Build history of the part. All positions in model axes, mm. A direction names the side the tool comes from. Coordinates: 2 decimals unless noted, no trailing zeros. Loops run counter-clockwise (first coordinate to the right, second up) from the corner with the lowest first, then second, coordinate; pieces in that order, holes last. Notation, with made-up numbers: (70, 23.5) -> (91, 23.5) arc R12 ccw to (91, 32.5) -> close; hole circle Ø4 at (38, 14.5). An arc over 180 degrees is marked (long way). One line per item, written item: value. Start each with the question number.
```python
from build123d import *

# Parameters (mm, degrees)
F0_W     = 55
F0_H     = 70
F1_DEPTH = 33
F2_T     = -3
F3_W     = 5
F3_H     = 30
F4_DEPTH = 55
F5_R     = 5.5
F6_DEPTH = 3
F7_R     = 1.65
F8_DEPTH = 3


with BuildPart() as f1:
    # F0 (on Top) → F1 (new body)
    with BuildSketch(Plane.XY):
        with Locations((27.5, 35)):
            Rectangle(F0_W, F0_H)
    extrude(amount=F1_DEPTH)

    # F2
    f2_openings = [f1.faces().sort_by_distance(p)[0] for p in [
        (27.5, 35, 0),
    ]]
    offset(amount=F2_T, openings=f2_openings)

    # F3 (on face) → F4 (cut, through all)
    with BuildSketch(Plane.YZ.offset(55)):
        with Locations((67.5, 15)):
            Rectangle(F3_W, F3_H)
    extrude(amount=-F4_DEPTH, mode=Mode.SUBTRACT)

    # F5 (on face) → F6 (cut, through all)
    with BuildSketch(Plane.XZ):
        with Locations((10, 11)):
            Circle(F5_R)
    extrude(amount=-F6_DEPTH, mode=Mode.SUBTRACT)

    # F7 (on face) → F8 (cut, through all)
    with BuildSketch(Plane.XY.offset(33)):
        with Locations((27.5, 67.5)):
            Circle(F7_R)
    extrude(amount=-F8_DEPTH, mode=Mode.SUBTRACT)


solid = f1.part
```
Item 1: Band-saw the part on D-D, the plane x = 43. List the corners of the cut face in (y, z).
Item 2: Tool access for faces 4 (the face through (27, 0, 16)), 5 (the face through (3, 34, 15)), 6 (the face through (54, 65, 15)): list every direction of +Z, -Z, +X, -X, +Y, -Y with a clear straight run to the whole face (end or side of a thin tool).
Item 3: Drop flat-ended pins along their axis: pin 1 Ø0.9 at (x, z) = (2, 18.5) entering from +Y; pin 2 Ø1 at (x, z) = (48, 15.5) entering from +Y; pin 3 Ø10 at (x, y) = (41.5, 40) entering from -Z. Give the stop position or say it passes through.
Item 4: Band-saw the part on C-C, the plane z = 17.5. List the corners of the cut face in (x, y), and give its area (3 significant figures).
Item 5: Probe probe 1 along X at (y, z) = (34, 4); probe 2 along Z at (x, y) = (10, 0.6); probe 3 along Z at (x, y) = (10, 10). List the from-to ranges inside material, lowest first.
Item 6: Band-saw the part on A-A, the plane x = 27.5. List the corners of the cut face in (y, z), and give its area (3 significant figures).
Item 7: Two-plate mould, pull along Y, no slides. Class faces 1 (the face through (27.1, 65.9, 31.5)), 2 (the face through (15.08, 1.48, 8.89)), 3 (the face through (2, 65, 15)): +Y half, -Y half, draft (parallel to the pull), parting line (faces both ways), or undercut.
Item 8: Band-saw the part on B-B, the plane y = 67.5. List the corners of the cut face in (x, z).
Worked out:
1. outline: (0, 0) -> (3, 0) -> (3, 30) -> (70, 30) -> (70, 33) -> (0, 33) -> close
2. face 4: +Z, -Z, +X, -X, -Y
2. face 5: -Z, +Y
2. face 6: -Z, +X, -X, +Y
3. pin 1: stops at y = 65
3. pin 2: stops at y = 3
3. pin 3: stops at z = 30
4. outline: (0, 0) -> (55, 0) -> (55, 65) -> (52, 65) -> (52, 3) -> (3, 3) -> (3, 65) -> (0, 65) -> close
4. area: 537 mm²
5. probe 1: x = 0 to 3, 52 to 55
5. probe 2: z = 0 to 5.5, 16.5 to 33
5. probe 3: z = 30 to 33
6. outline: (0, 0) -> (3, 0) -> (3, 30) -> (65.85, 30) -> (65.85, 33) -> (0, 33) -> close; (69.15, 30) -> (70, 30) -> (70, 33) -> (69.15, 33) -> close
6. area: 290 mm²
7. face 1: undercut
7. face 2: draft
7. face 3: +Y half
8. outline: (0, 30) -> (25.85, 30) -> (25.85, 33) -> (0, 33) -> close; (29.15, 30) -> (55, 30) -> (55, 33) -> (29.15, 33) -> close
